Verification items for the finished model (mm, model axes). A direction names the side the tool comes from. Coordinates: 2 decimals unless noted, no trailing zeros. Write each loop counter-clockwise with the first axis right and the second up, starting at its lowest first coordinate (ties: lowest second). Pieces come first, ordered by that corner, then holes. Notation, with made-up numbers: (80.5, -36) -> (122.5, -36) arc R29 cw to (122.5, -7) -> close; hole circle Ø9 at (16.5, 82). An arc over 180 degrees is marked (long way). Write item = value, one per line. Start each with the question number.
(1) Section check B-B (x = 0). Record the cut outline in (y, z).
(2) Section check A-A (z = 0). Record the cut outline in (x, y).
(3) Mould release check, pull along Y, two halves, no side actions. Record for faces 1 (the face through (1, 149, 3)), 2 (the face through (0.9, 151.97, 2.86)), 3 (the face through (0, 170, 0)): released by +Y, released by -Y, zero draft, split by the parting line, or undercut.
(4) Section check C-C (y = 60). Record the cut outline in (x, z), plus the area to 3 significant figures.
(5) Gauge pin test, flat ends, axial feed: pin 1 Ø1.5 at (x, y) = (2, 23.5) entering from +Z; pin 2 Ø5 at (y, z) = (90, -3.5) entering from +X; pin 3 Ø3 at (x, y) = (1.5, 149.5) entering from -Z. Record the tip position at first contact, or that the pin passes through.
(6) Material ranges on probe 1 along Y at (x, z) = (-4, 0.25); probe 2 along Y at (x, z) = (2.5, -1.75); probe 3 along X at (y, z) = (125, 0.25), recorded low to high. Write a range as [from, to].
(7) Set-up check for faces 4 (the face through (1, 150, 3)), 5 (the face through (0.9, 73.46, 2.86)), 6 (the face through (1.352, -4.93, -4.292)): record each of +Z, -Z, +X, -X, +Y, -Y from which the full face is reachable in a straight line by a thin tool's end or side.
```python
from build123d import *

# Parameters (mm, degrees)
SKETCH2_R           = 3
BOSS_EXTRUDE1_DEPTH = 170
SKETCH3_R           = 4.5
BOSS_EXTRUDE2_DEPTH = 10
SKETCH4_OUTSIDE_W   = 47.09
SKETCH4_OUTSIDE_H   = 47.09
SKETCH4_OUTSIDE_R   = 2.75
CUT_EXTRUDE1_DEPTH  = 16
BOSS_EXTRUDE3_START = -21
SKETCH5_R           = 3.5
BOSS_EXTRUDE3_DEPTH = 1


with BuildPart() as part:
    # Sketch2 → Boss-Extrude1 (new body)
    with BuildSketch(Plane(origin=(0, 0, 0), x_dir=(1, 0, 0), z_dir=(0, 1, 0))):
        with Locations(Location((0, 0, 0), (0, 0, 270))):  # turned: the seam where the file's is
            Circle(SKETCH2_R)
    extrude(amount=BOSS_EXTRUDE1_DEPTH)

    # Sketch3 → Boss-Extrude2 (add)
    with BuildSketch(Plane.XZ):
        with Locations(Location((0, 0, 0), (0, 0, 270))):  # turned: the seam where the file's is
            Circle(SKETCH3_R)
    extrude(amount=BOSS_EXTRUDE2_DEPTH)

    # Sketch4 outside → Cut-Extrude1 (cut)
    with BuildSketch(Plane(origin=(0, 170, 0), x_dir=(1, 0, 0), z_dir=(0, 1, 0))):
        Rectangle(SKETCH4_OUTSIDE_W, SKETCH4_OUTSIDE_H)
        with Locations(Location((0, 0, 0), (0, 0, 270))):  # turned: the seam where the file's is
            Circle(SKETCH4_OUTSIDE_R, mode=Mode.SUBTRACT)
    extrude(amount=-CUT_EXTRUDE1_DEPTH, mode=Mode.SUBTRACT)

    # Sketch5 → Boss-Extrude3 (add)
    with BuildSketch(Plane(origin=(0, 170, 0), x_dir=(1, 0, 0), z_dir=(0, 1, 0)).offset(BOSS_EXTRUDE3_START)):
        with Locations(Location((0, 0, 0), (0, 0, 270))):  # turned: the seam where the file's is
            Circle(SKETCH5_R)
    extrude(amount=BOSS_EXTRUDE3_DEPTH)


solid = part.part
```
Response:
q1.outline = (-10, -4.5) -> (0, -4.5) -> (0, -3) -> (149, -3) -> (149, -3.5) -> (150, -3.5) -> (150, -3) -> (154, -3) -> (154, -2.75) -> (170, -2.75) -> (170, 2.75) -> (154, 2.75) -> (154, 3) -> (150, 3) -> (150, 3.5) -> (149, 3.5) -> (149, 3) -> (0, 3) -> (0, 4.5) -> (-10, 4.5) -> close
q2.outline = (-4.5, -10) -> (4.5, -10) -> (4.5, 0) -> (3, 0) -> (3, 149) -> (3.5, 149) -> (3.5, 150) -> (3, 150) -> (3, 154) -> (2.75, 154) -> (2.75, 170) -> (-2.75, 170) -> (-2.75, 154) -> (-3, 154) -> (-3, 150) -> (-3.5, 150) -> (-3.5, 149) -> (-3, 149) -> (-3, 0) -> (-4.5, 0) -> close
q3.face_1 = undercut
q3.face_2 = zero draft
q3.face_3 = released by +Y
q4.outline = circle Ø6 at (0, 0)
q4.area = 28.3 mm2
q5.pin_1 = 2.73
q5.pin_2 = 2.83
q5.pin_3 = -3.5
q6.probe_1 = [-10, 0]
q6.probe_2 = [-10, 0], [149, 150]
q6.probe_3 = [-2.99, 2.99]
q7.face_4 = +Y
q7.face_5 = none
q7.face_6 = +Y, -Y
